```python
from build123d import *

# Parameters (mm, degrees)
F1_ANGLE_BACK   = 45
F1_ANGLE        = 180
F2_SIZE         = 1
F4_D            = 6.6
F4_CSINK_D      = 13.44
F4_CSINK_ANGLE  = 90
F6_DEPTH        = 40
F8_DEPTH        = 50
F12_D           = 5.5
F12_CBORE_D     = 9.75
F12_CBORE_DEPTH = 5


# Not quite as in the source:
# - a feature names something its author has since deleted; it is built from what else it names


with BuildPart() as f1:
    # F0 (on Front) → F1 (revolve)
    with BuildSketch(Plane.XZ, mode=Mode.PRIVATE) as f1_sk:
        Polygon((0, 10), (0, 0), (31.6, 0), (31.6, -7), (37.5, -7), (37.5, 10), align=None)
    revolve(f1_sk.sketch.rotate(Axis((0, 0, 5), (0, 0, -1)), -F1_ANGLE_BACK), axis=Axis((0, 0, 5), (0, 0, -1)), revolution_arc=F1_ANGLE)

    # F2
    f2_edges = [f1.edges().sort_by_distance(p)[0] for p in [
        (22.344574, -22.344574, -7),
        (26.516504, -26.516504, -7),
        (26.516504, -26.516504, 10),
    ]]
    chamfer(f2_edges, length=F2_SIZE)

    # F4 (through all)
    with Locations(Plane.XY.offset(10)):
        with Locations((25, 0), (0, -25)):
            CounterSinkHole(F4_D / 2, F4_CSINK_D / 2, counter_sink_angle=F4_CSINK_ANGLE)

    # F5 (on face) → F6 (join)
    with BuildSketch(Plane.XY.offset(10)):
        with BuildLine():
            Line((19.4820004924, 5.3398648686), (7.0710678119, -7.0710678119))
            Line((7.0710678119, -7.0710678119), (-5.3398648686, -19.4820004924))
            ThreePointArc((-5.3398648686, -19.4820004924), (0.79408889, -17.1167209324), (7.0710678119, -19.0710678119))
            ThreePointArc((7.0710678119, -19.0710678119), (19.0710678119, -19.0710678119), (19.0710678119, -7.0710678119))
            ThreePointArc((19.0710678119, -7.0710678119), (17.1167209324, -0.79408889), (19.4820004924, 5.3398648686))
        make_face()
        with BuildLine():
            Line((7.0710678119, -7.0710678119), (0, 0))
            Line((0, 0), (-25.8093975133, -25.8093975133))
            ThreePointArc((-25.8093975133, -25.8093975133), (-21.9914756212, -29.1311688746), (-17.7507975491, -31.8929331729))
            Line((-17.7507975491, -31.8929331729), (-5.3398648686, -19.4820004924))
            Line((-5.3398648686, -19.4820004924), (7.0710678119, -7.0710678119))
        make_face()
        with BuildLine():
            Line((25.8093975133, 25.8093975133), (0, 0))
            Line((0, 0), (7.0710678119, -7.0710678119))
            Line((7.0710678119, -7.0710678119), (19.4820004924, 5.3398648686))
            Line((19.4820004924, 5.3398648686), (31.8929331729, 17.7507975491))
            ThreePointArc((31.8929331729, 17.7507975491), (29.1311688746, 21.9914756212), (25.8093975133, 25.8093975133))
        make_face()
    extrude(amount=F6_DEPTH)

    # F7 (on face) → F8 (join)
    with BuildSketch(Plane.XY.offset(50)):
        with BuildLine():
            ThreePointArc((36.4612769111, -1.6808587126), (35.531279534, 8.3533331479), (31.8929331729, 17.7507975491))
            Line((31.8929331729, 17.7507975491), (19.4820004924, 5.3398648686))
            ThreePointArc((19.4820004924, 5.3398648686), (17.1167209324, -0.79408889), (19.0710678119, -7.0710678119))
            ThreePointArc((19.0710678119, -7.0710678119), (21.5563491861, -13.0710678119), (19.0710678119, -19.0710678119))
            Line((19.0710678119, -19.0710678119), (36.4612769111, -1.6808587126))
        make_face()
        with BuildLine():
            Line((-5.3398648686, -19.4820004924), (-17.7507975491, -31.8929331729))
            ThreePointArc((-17.7507975491, -31.8929331729), (-8.3533331479, -35.531279534), (1.6808587126, -36.4612769111))
            Line((1.6808587126, -36.4612769111), (19.0710678119, -19.0710678119))
            ThreePointArc((19.0710678119, -19.0710678119), (13.0710678119, -21.5563491861), (7.0710678119, -19.0710678119))
            ThreePointArc((7.0710678119, -19.0710678119), (0.79408889, -17.1167209324), (-5.3398648686, -19.4820004924))
        make_face()
        with BuildLine():
            ThreePointArc((31.8929331729, 17.7507975491), (29.1311688746, 21.9914756212), (25.8093975133, 25.8093975133))
            Line((25.8093975133, 25.8093975133), (-25.8093975133, -25.8093975133))
            ThreePointArc((-25.8093975133, -25.8093975133), (-21.9914756212, -29.1311688746), (-17.7507975491, -31.8929331729))
            Line((-17.7507975491, -31.8929331729), (-5.3398648686, -19.4820004924))
            ThreePointArc((-5.3398648686, -19.4820004924), (0.79408889, -17.1167209324), (7.0710678119, -19.0710678119))
            ThreePointArc((7.0710678119, -19.0710678119), (13.0710678119, -21.5563491861), (19.0710678119, -19.0710678119))
            ThreePointArc((19.0710678119, -19.0710678119), (21.5563491861, -13.0710678119), (19.0710678119, -7.0710678119))
            ThreePointArc((19.0710678119, -7.0710678119), (17.1167209324, -0.79408889), (19.4820004924, 5.3398648686))
            Line((19.4820004924, 5.3398648686), (31.8929331729, 17.7507975491))
        make_face()
    extrude(amount=F8_DEPTH)

    # F9 (on face) → F10 (revolve, cut)
    with BuildSketch(Plane(origin=(0, 0, 0), x_dir=(-0.7071067812, -0.7071067812, 0), z_dir=(-0.7071067812, 0.7071067812, 0))):
        Polygon((36.5, 86.5), (-36.5, 85.5), (-36.5, 75), (36.5, 75), align=None)
    revolve(axis=Axis((0, 0, 75), (-0.7071067812, -0.7071067812, 0)), mode=Mode.SUBTRACT)

    # F12 (through all)
    with Locations(Plane(origin=(19.0710678119, -19.0710678119, 0), x_dir=(0.7071067812, 0.7071067812, 0), z_dir=(0.7071067812, -0.7071067812, 0))):
        with Locations((20.5934695606, 93.5), (20.5934695606, 56.5), (-20.5934695606, 56.5), (-20.5934695606, 93.5)):
            CounterBoreHole(F12_D / 2, F12_CBORE_D / 2, F12_CBORE_DEPTH)


solid = f1.part
```
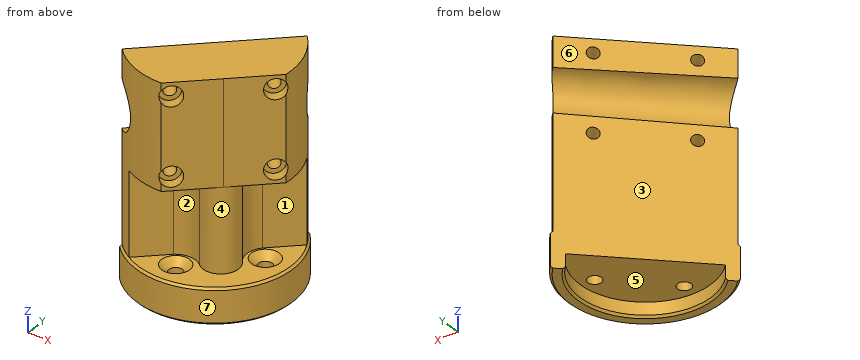
Here's how the part is built. I have some questions about the finished solid (model axes, mm). Face numbers are marked on the shaded views. A direction names the side the tool comes from. Round coordinates to 2 decimals unless told otherwise and drop trailing zeros. Loops run counter-clockwise (first coordinate to the right, second up) from the corner with the lowest first, then second, coordinate; pieces in that order, holes last.
1. Thinking about a two-plate mould opening in Y: for the marked faces 5, 6 and 7, which applies, released by +Y, released by -Y, zero draft, split by the parting line, or undercut?
Answers:
face 5: undercut
face 6: released by +Y
face 7: split by the parting line
2. For the marked faces 1, 2, 3 and 4, which set-ups out of +Z, -Z, +X, -X, +Y, -Y let a thin tool reach every point of the face, with its end or its side?
Answers:
face 1: +X
face 2: -Y
face 3: +Z, -Z, -X, +Y
face 4: none
3. Will these pins go through, and if not, where does the flat tip stop? pin 1 (7.5 mm diameter, centred on x = 0, y = -25, fed in from -Z); pin 2 (1 mm diameter, centred on x = -17.5, z = 24.5, fed in from -Y); pin 3 (10 mm diameter, centred on x = 11.5, z = 52.5, fed in from +Y); pin 4 (10 mm diameter, centred on x = -10, y = -1.5, fed in from +Z).
Answers:
pin 1: stops at z = 0
pin 2: stops at y = -31.89
pin 3: stops at y = 16.5
pin 4: passes through
4. Suppose I cut it at A-A, the plane z = 22.5. Please give me the cut outline in (x, y).
Answers:
outline: (-25.81, -25.81) arc R36.5 ccw to (-17.75, -31.89) - (-5.34, -19.48) arc R10 cw to (7.07, -19.07) arc R8.49 ccw to (19.07, -7.07) arc R10 cw to (19.48, 5.34) - (31.89, 17.75) arc R36.5 ccw to (25.81, 25.81) - close
5. If I drill on probe 1 along Y at (x, z) = (0, 4); probe 2 along Z at (x, y) = (9, -26.5); probe 3 along Z at (x, y) = (-14, -16), over which ranges is the centre line in solid material (lowest first)?
Answers:
probe 1: y = -37.5 to -28.3, -21.7 to 0
probe 2: z = 0 to 10, 50 to 100
probe 3: z = 0 to 53.82, 59.18 to 63.8, 86.2 to 90.82, 96.18 to 100
